```python
from build123d import *

# Parameters (mm, degrees)
BOSS_EXTRUDE1_DEPTH = 3.175
FILLET2_R           = 40
FILLET3_R           = 20
SKETCH2_R           = 2.1
CUT_EXTRUDE1_DEPTH  = 129.167166232
SKETCH3_R           = 2.1
CUT_EXTRUDE2_DEPTH  = 129.167166232
SKETCH4_R           = 2.1
CUT_EXTRUDE3_DEPTH  = 129.167166232


with BuildPart() as part:
    # Sketch1 → Boss-Extrude1 (new, symmetric)
    with BuildSketch(Plane.XY):
        Polygon((-69.5, 107.5), (-69.5, 43.5), (5.5, 43.5), (5.5, -107.5), (69.5, -107.5), (69.5, 107.5), align=None)
    extrude(amount=BOSS_EXTRUDE1_DEPTH, both=True)

    # Fillet2
    fillet2_edges = [part.edges().sort_by_distance(p)[0] for p in [
        (69.5, 107.5, 0),
    ]]
    fillet(fillet2_edges, radius=FILLET2_R)

    # Fillet3
    fillet3_edges = [part.edges().sort_by_distance(p)[0] for p in [
        (5.5, 43.5, 0),
    ]]
    fillet(fillet3_edges, radius=FILLET3_R)

    # Sketch2 → Cut-Extrude1 (cut, through all)
    with BuildSketch(Plane.XY.offset(3.175)):
        with Locations((-37.5, 101.15)):
            Circle(SKETCH2_R)
        with Locations((-51.5, 101.15)):
            Circle(SKETCH2_R)
        with Locations((-65.5, 101.15)):
            Circle(SKETCH2_R)
        with Locations((-65.5, 46.675)):
            Circle(SKETCH2_R)
        with Locations((-37.5, 46.675)):
            Circle(SKETCH2_R)
        with Locations((-51.5, 46.675)):
            Circle(SKETCH2_R)
    extrude(amount=-CUT_EXTRUDE1_DEPTH, mode=Mode.SUBTRACT)

    # Sketch3 → Cut-Extrude2 (cut, through all)
    with BuildSketch(Plane.XY.offset(3.175)):
        with Locations((66.325, -92)):
            Circle(SKETCH3_R)
        with Locations((66.325, 52)):
            Circle(SKETCH3_R)
        with Locations((66.325, -20)):
            Circle(SKETCH3_R)
    extrude(amount=-CUT_EXTRUDE2_DEPTH, mode=Mode.SUBTRACT)

    # Sketch4 → Cut-Extrude3 (cut, through all)
    with BuildSketch(Plane.XY.offset(3.175)):
        with Locations((8.675, -96)):
            Circle(SKETCH4_R)
        with Locations((8.675, -42)):
            Circle(SKETCH4_R)
        with Locations((8.675, 12)):
            Circle(SKETCH4_R)
    extrude(amount=-CUT_EXTRUDE3_DEPTH, mode=Mode.SUBTRACT)


solid = part.part
```
The listing builds one solid part. Answer for the finished solid, in the listing's coordinates (mm). Give positions to 0.01 mm unless a question says otherwise; leave off trailing zeros. Order: outer loops, then holes, each group sorted by start corner. A loop starts at its lowest first (then second) coordinate and runs counter-clockwise, first axis right, second up. Notation, with made-up numbers: (35.5, 4.5) -> (46.5, 4.5) arc R18 ccw to (46.5, 16.5) -> close; hole circle Ø10 at (-38.75, 2). An arc over 180 degrees is marked (long way). Answer as CSV lines item,"result". Start each with the question number.
Q1. A cutting plane is placed at A-A (y = -20). Determine the outline of the cut face in (x, z) (3 decimals), then the cut area to 3 significant figures.
Q2. Given pin 1 (3.5 mm diameter, centred on x = -37.5, y = 101.15, fed in from +Z), flat-ended and moving along its own axis, determine where the tip first touches the part or whether it passes through.
Q3. Find the intervals of material crossed by L1, parallel to Y at x = -65.5, z = 1.5 (3 decimals); L2, parallel to X at y = 1.5, z = 2.25; L3, parallel to Y at x = -40, z = 0.75, in increasing order.
Q4. A cutting plane is placed at D-D (z = 1.75). Count the separate pieces of the cut face and the enclosed holes in it, then the cut area to 3 significant figures.
Q5. A cutting plane is placed at B-B (x = -51.5). Determine the outline of the cut face in (y, z) (3 decimals).
Q6. Determine the mould class of faces 1 (the flat face through (69.5, -21, 0)), 2 (the cylindrical face through (-37.96, 99.1, 0.04)), 3 (the flat face through (14, 25, -3.175)) for opening direction X: pulls with the +X half, pulls with the -X half, needs draft (parallel to the pull), parting line crosses it, or undercut.
Q7. A cutting plane is placed at C-C (y = 52). Determine the outline of the cut face in (x, z) (3 decimals).
Results found:
1,outline,"(5.5, -3.175) -> (64.225, -3.175) -> (64.225, 3.175) -> (5.5, 3.175) -> close; (68.425, -3.175) -> (69.5, -3.175) -> (69.5, 3.175) -> (68.425, 3.175) -> close"
1,area,"380 mm2"
2,pin 1,"through"
3,L1,"43.5 to 44.575, 48.775 to 99.05, 103.25 to 107.5"
3,L2,"5.5 to 69.5"
3,L3,"43.5 to 107.5"
4,separate pieces,"1"
4,enclosed holes,"12"
4,area,"18,100 mm2"
5,outline,"(43.5, -3.175) -> (44.575, -3.175) -> (44.575, 3.175) -> (43.5, 3.175) -> close; (48.775, -3.175) -> (99.05, -3.175) -> (99.05, 3.175) -> (48.775, 3.175) -> close; (103.25, -3.175) -> (107.5, -3.175) -> (107.5, 3.175) -> (103.25, 3.175) -> close"
6,face 1,"pulls with the +X half"
6,face 2,"undercut"
6,face 3,"needs draft"
7,outline,"(-69.5, -3.175) -> (64.225, -3.175) -> (64.225, 3.175) -> (-69.5, 3.175) -> close; (68.425, -3.175) -> (69.5, -3.175) -> (69.5, 3.175) -> (68.425, 3.175) -> close"
